Source: CAD feature listing. Evaluate the final solid. Frame: model axes, mm. A direction names the side the tool comes from. Coordinates: 2 decimals unless noted, no trailing zeros. Write each loop counter-clockwise with the first axis right and the second up, starting at its lowest first coordinate (ties: lowest second). Pieces come first, ordered by that corner, then holes. Notation, with made-up numbers: M 13.25,53 L 35.25,53 A34 cw 35.25,84 Z; hole C -0.5,-2.5 d6. An arc over 180 degrees is marked long. Write item = value, one per line. Start each with the question number.
1. Line query: line 1 along X through (y, z) = (113, 18.25); line 2 along Z through (x, y) = (653, 133.5); line 3 along X through (y, z) = (211.5, 6.75). Output: solid intervals per line, ascending.
2. Section query B-B (y = 154). Output: boundary loops of the cut face in (x, z).
3. Section query A-A (y = 193). Output: boundary loops of the cut face in (x, z).
4. Pull-direction query (Z, two-part tool) for faces 5 (the face through (607.35, 226, 14)), 6 (the face through (647, 217.5, 11)), 7 (the face through (594, 167, 25)), 8 (the face through (594.71, 221.18, 26.52)); classes: pulls with the +Z half, pulls with the -Z half, needs draft (parallel to the pull), parting line crosses it, or undercut.
5. Pin query (flat end, axial travel): pin 1 Ø1.5 at (x, z) = (639.5, 16) entering from -Y; pin 2 Ø7.5 at (y, z) = (176, 14.5) entering from +X; pin 3 Ø16 at (x, y) = (697, 192.5) entering from -Z; pin 4 Ø5 at (y, z) = (138, 7.5) entering from -X. Return the tip coordinate at first contact, or that it passes through.
6. Section query C-C (x = 668). Output: boundary loops of the cut face in (y, z), then the cut area to 4 significant figures.
7. Access query for faces 1 (the face through (694.3, 162, 12)), 2 (the face through (601.81, 231.09, 12.68)), 3 (the face through (689.944, 159.572, 23.934)), 4 (the face through (648, 226, 8)). Directions: +Z, -Z, +X, -X, +Y, -Y. A direction counts if a zero-diameter tool reaches every point of the face in a straight line with its end or side. Return the directions, or none.
8. Section query D-D (z = 4.5). Output: boundary loops of the cut face in (x, y), then the cut area to 3 significant figures.
```python
from build123d import *

# Parameters (mm, degrees)
SKETCH154_W      = 94.3
SKETCH154_H      = 133
PAD011_DEPTH     = 28
SKETCH155_W      = 91
SKETCH155_H      = 25
POCKET032_DEPTH  = 117.5
FILLET010_R      = 9
FILLET011_R      = 5
SKETCH157_W      = 133
SKETCH157_H      = 3
PAD012_DEPTH     = 8
SKETCH158_W      = 133
SKETCH158_H      = 3
PAD013_DEPTH     = 8
FILLET012_R      = 6.35
SKETCH159_W      = 79.65001
SKETCH159_H      = 12
POCKET033_DEPTH  = 14
SKETCH160_W      = 18.3
SKETCH160_H      = 4.3
POCKET034_DEPTH  = 2
FILLET013_R      = 2
SKETCH164_R      = 1.75
POCKET037_DEPTH  = 3
FILLET017_R      = 3
FILLET018_R      = 1
HOLE_D           = 3.5
HOLE_DEPTH       = 25
HOLE_CSINK_D     = 6.1
HOLE_CSINK_ANGLE = 90


with BuildPart() as part:
    # Sketch154 → Pad011 (new body)
    with BuildSketch(Plane.XY):
        with Locations((647.15, 166.5)):
            Rectangle(SKETCH154_W, SKETCH154_H)
    extrude(amount=PAD011_DEPTH)

    # Sketch155 (on Face1 of Pad011) → Pocket032 (cut)
    with BuildSketch(Plane.XZ.offset(-100)):
        with Locations((647.149987, 13.999999)):
            Rectangle(SKETCH155_W, SKETCH155_H)
    extrude(amount=-POCKET032_DEPTH, mode=Mode.SUBTRACT)

    # Fillet010
    fillet010_edges = [part.edges().sort_by_distance(p)[0] for p in [
        (692.649987, 158.75, 26.499999),
        (601.649987, 158.75, 26.499999),
    ]]
    fillet(fillet010_edges, radius=FILLET010_R)

    # Fillet011
    fillet011_edges = [part.edges().sort_by_distance(p)[0] for p in [
        (601.649987, 158.75, 1.499999),
        (692.649987, 158.75, 1.499999),
    ]]
    fillet(fillet011_edges, radius=FILLET011_R)

    # Sketch157 (on Face13 of Fillet011) → Pad012 (join)
    with BuildSketch(Plane.YZ.offset(694.3)):
        with Locations((166.5, 26.5)):
            Rectangle(SKETCH157_W, SKETCH157_H)
    extrude(amount=PAD012_DEPTH)

    # Sketch158 (on Face10 of Pad012) → Pad013 (join)
    with BuildSketch(Plane(origin=(600, 0, 0), x_dir=(0, -1, 0), z_dir=(-1, 0, 0))):
        with Locations((-166.500003, 26.5)):
            Rectangle(SKETCH158_W, SKETCH158_H)
    extrude(amount=PAD013_DEPTH)

    # Fillet012
    fillet012_edges = [part.edges().sort_by_distance(p)[0] for p in [
        (600, 233, 12.5),
        (694.3, 233, 12.5),
        (702.3, 233, 26.5),
        (592, 233.000003, 26.5),
    ]]
    fillet(fillet012_edges, radius=FILLET012_R)

    # Sketch159 (on Face10 of Fillet012) → Pocket033 (cut)
    with BuildSketch(Plane(origin=(0, 233, 0), x_dir=(-1, 0, 0), z_dir=(0, 1, 0))):
        with Locations((-647.174991, 14)):
            Rectangle(SKETCH159_W, SKETCH159_H)
    extrude(amount=-POCKET033_DEPTH, mode=Mode.SUBTRACT)

    # Sketch160 (on Face35 of Pocket033) → Pocket034 (cut)
    with BuildSketch(Plane(origin=(0, 219, 0), x_dir=(-1, 0, 0), z_dir=(0, 1, 0))):
        with Locations((-647.199985, 14.05)):
            Rectangle(SKETCH160_W, SKETCH160_H)
    extrude(amount=-POCKET034_DEPTH, mode=Mode.SUBTRACT)

    # Fillet013
    fillet013_edges = [part.edges().sort_by_distance(p)[0] for p in [
        (638.049985, 218.25, 11.9),
        (638.049985, 218.25, 16.2),
        (656.349985, 218.25, 16.2),
        (656.349985, 218.25, 11.9),
    ]]
    fillet(fillet013_edges, radius=FILLET013_R)

    # Sketch164 (on Face26 of Fillet013) → Pocket037 (cut)
    with BuildSketch(Plane.XY.offset(28)):
        with Locations((698.30001, 111.85331)):
            Circle(SKETCH164_R)
        with Locations((596, 111.85331)):
            Circle(SKETCH164_R)
        with Locations((596, 139.168671)):
            Circle(SKETCH164_R)
        with Locations((698.30001, 139.168671)):
            Circle(SKETCH164_R)
        with Locations((698.30001, 166.000002)):
            Circle(SKETCH164_R)
        with Locations((698.30001, 193)):
            Circle(SKETCH164_R)
        with Locations((698.30001, 219.999573)):
            Circle(SKETCH164_R)
        with Locations((596, 219.999573)):
            Circle(SKETCH164_R)
        with Locations((596, 193)):
            Circle(SKETCH164_R)
        with Locations((596, 166)):
            Circle(SKETCH164_R)
    extrude(amount=-POCKET037_DEPTH, mode=Mode.SUBTRACT)

    # Fillet017
    fillet017_edges = [part.edges().sort_by_distance(p)[0] for p in [
        (592, 100.000003, 26.5),
        (702.3, 100, 26.5),
    ]]
    fillet(fillet017_edges, radius=FILLET017_R)

    # Fillet018
    fillet018_edges = [part.edges().sort_by_distance(p)[0] for p in [
        (607.349986, 226, 20),
        (607.349986, 226, 8),
        (686.999996, 226, 8),
        (686.999996, 226, 20),
    ]]
    fillet(fillet018_edges, radius=FILLET018_R)

    # Hole
    with Locations(Plane.XY.offset(1.499999)):
        with Locations((621.615906, 112), (673.700684, 112)):
            CounterSinkHole(HOLE_D / 2, HOLE_CSINK_D / 2, depth=HOLE_DEPTH, counter_sink_angle=HOLE_CSINK_ANGLE)


solid = part.part
```
Results are:
q1.line_1 = 600 to 601.68, 692.62 to 694.3
q1.line_2 = 0 to 1.5, 26.5 to 28
q1.line_3 = 600 to 601.65, 692.65 to 694.3
q2.outline = M 592,25 L 600,25 L 600,0 L 694.3,0 L 694.3,25 L 702.3,25 L 702.3,28 L 592,28 Z; hole M 601.65,6.5 A5 ccw 606.65,1.5 L 687.65,1.5 A5 ccw 692.65,6.5 L 692.65,17.5 A9 ccw 683.65,26.5 L 610.65,26.5 A9 ccw 601.65,17.5 Z
q3.outline = M 592,25 L 594.25,25 L 594.25,28 L 592,28 Z; M 597.75,25 L 600,25 L 600,0 L 694.3,0 L 694.3,25 L 696.55,25 L 696.55,28 L 597.75,28 Z; M 700.05,25 L 702.3,25 L 702.3,28 L 700.05,28 Z; hole M 601.65,6.5 A5 ccw 606.65,1.5 L 687.65,1.5 A5 ccw 692.65,6.5 L 692.65,17.5 A9 ccw 683.65,26.5 L 610.65,26.5 A9 ccw 601.65,17.5 Z
q4.face_5 = undercut
q4.face_6 = undercut
q4.face_7 = pulls with the -Z half
q4.face_8 = needs draft
q5.pin_1 = 217.5
q5.pin_2 = 694.3
q5.pin_3 = 0
q5.pin_4 = 600
q6.outline = M 100,0 L 233,0 L 233,8 L 219,8 L 219,20 L 233,20 L 233,28 L 100,28 L 100,26.5 L 217.5,26.5 L 217.5,1.5 L 100,1.5 Z
q6.area = 618.5 mm^2
q7.face_1 = -Z, +X, +Y, -Y
q7.face_2 = -Z, -X, +Y
q7.face_3 = -Y
q7.face_4 = +Y
q8.outline = M 600,100 L 602.07,100 L 602.07,217.5 L 692.23,217.5 L 692.23,100 L 694.3,100 L 694.3,226.65 A6.35 ccw 687.95,233 L 606.35,233 A6.35 ccw 600,226.65 Z
q8.area = 1,930 mm^2
